For this review, take the finished solid that the model builds, in its own axes (mm). A direction names the side the tool comes from. Give positions to 0.01 mm unless a question says otherwise; leave off trailing zeros. Loops run counter-clockwise (first coordinate to the right, second up) from the corner with the lowest first, then second, coordinate; pieces in that order, holes last. Notation, with made-up numbers: (-36.75, 5.5) - (-9.75, 5.5) arc R20 ccw to (-9.75, 14.5) - close; hole circle Ø5 at (77.5, -19.75). An arc over 180 degrees is marked (long way). Answer in a Markdown table with one row per item.
```python
from build123d import *

# Parameters (mm, degrees)
F1_DEPTH = 22
F2_R     = 4
F3_DEPTH = 18.579489


with BuildPart() as f1:
    # F0 (on Front) → F1 (new body)
    with BuildSketch(Plane.XZ):
        with BuildLine():
            ThreePointArc((3.232615, 2.016507), (-0.015975, -3.809967), (-3.215592, 2.043544))
            Line((-3.215592, 2.043544), (-3.215592, 16.849984))
            Line((-3.215592, 16.849984), (-9.248437, 16.849984))
            Line((-9.248437, 16.849984), (-9.248437, 3.271468))
            ThreePointArc((-9.248437, 3.271468), (-0.128645, -9.809156), (9.331051, 3.027802))
            Line((9.331051, 3.027802), (9.331051, 16.849984))
            Line((9.331051, 16.849984), (3.232615, 16.849984))
            Line((3.232615, 16.849984), (3.232615, 2.016507))
        make_face()
    extrude(amount=F1_DEPTH)

    # F2 (on face) → F3 (cut, through all)
    with BuildSketch(Plane.YZ.offset(9.331051)):
        with Locations((-11.015, 10.309984)):
            Circle(F2_R)
    extrude(amount=-F3_DEPTH, mode=Mode.SUBTRACT)


solid = f1.part
```
1. For faces 1 (the face through (-3.216, -11, 6)), 2 (the face through (-4, -22, 4)), 3 (the face through (-9.248, -8, 7)), list the 3-axis set-ups (+Z, -Z, +X, -X, +Y, -Y) from which the entire face can be reached by the end or side of a thin tool; tool diameter is ignored.
Values:
| item | result |
|---|---|
| face 1 | +Z, +Y, -Y |
| face 2 | +Z, -Z, +X, -X, -Y |
| face 3 | +Z, -X, +Y, -Y |
2. We need section A-A, the plane z = 15. Give the boundary of the cut face in (x, y).
Values:
| item | result |
|---|---|
| outline | (-9.25, -22) - (-3.22, -22) - (-3.22, 0) - (-9.25, 0) - close; (3.23, -22) - (9.33, -22) - (9.33, 0) - (3.23, 0) - close |
3. We need section C-C, the plane x = 0. Give the boundary of the cut face in (y, z).
Values:
| item | result |
|---|---|
| outline | (-22, -9.81) - (0, -9.81) - (0, -3.81) - (-22, -3.81) - close |
4. Clearance check with flat-ended pins moving along their axes: pin 1 (13 mm diameter, centred on y = -11.02, z = 10.31, fed in from -X); pin 2 (1 mm diameter, centred on x = 7, y = -18, fed in from -Z); pin 3 (1 mm diameter, centred on y = -18.5, z = 7.5, fed in from +X). State where each tip first meets the part, or that it passes through.
Values:
| item | result |
|---|---|
| pin 1 | stops at x = -9.25 |
| pin 2 | stops at z = -7.35 |
| pin 3 | stops at x = 9.33 |
5. Wall thickness on line 1 (X direction, y = -18.25, z = 15.75); line 2 (X direction, y = -11.5, z = 0.25); line 3 (Y direction, x = 8.5, z = 12.75): over which ranges is each line inside the solid? List them lowest first. Write a range as [from, to].
Values:
| item | result |
|---|---|
| line 1 | x = [-9.25, -3.22], [3.23, 9.33] |
| line 2 | x = [-9.81, -3.8], [3.8, 9.81] |
| line 3 | y = [-22, -14.18], [-7.85, 0] |
6. Mouldability with a two-part tool opening along X and no side actions: class faces 4 (the face through (9.331, -8, 7)), 5 (the face through (3.233, -11, 6)), 6 (the face through (-4, 0, 4)) as released by +X, released by -X, zero draft, split by the parting line, or undercut.
Values:
| item | result |
|---|---|
| face 4 | released by +X |
| face 5 | undercut |
| face 6 | zero draft |
7. We need section B-B, the plane y = -2.5. Give the boundary of the cut face in (x, z).
Values:
| item | result |
|---|---|
| outline | (-9.25, 3.27) arc R9.81 ccw (long way) to (9.33, 3.03) - (9.33, 16.85) - (3.23, 16.85) - (3.23, 2.02) arc R3.81 cw (long way) to (-3.22, 2.04) - (-3.22, 16.85) - (-9.25, 16.85) - close |
8. We need section D-D, the plane z = -1.5. Give the boundary of the cut face in (x, y).
Values:
| item | result |
|---|---|
| outline | (-9.69, -22) - (-3.5, -22) - (-3.5, 0) - (-9.69, 0) - close; (3.5, -22) - (9.69, -22) - (9.69, 0) - (3.5, 0) - close |
